```python
from build123d import *

# Parameters (mm, degrees)
SKETCH1_R           = 2.0828
SKETCH1_R_2         = 14.2875
SKETCH1_R_3         = 2.4892
BOSS_EXTRUDE1_DEPTH = 6.35


with BuildPart() as part:
    # Sketch1 → Boss-Extrude1 (new body)
    with BuildSketch(Plane(origin=(95.25, 0, 0), x_dir=(0, 0, -1), z_dir=(1, 0, 0))):
        with BuildLine():
            Line((-184.15, -107.95), (-184.15, -25.4))
            ThreePointArc((-184.15, -25.4), (-186.009871939, -20.909871939), (-190.5, -19.05))
            Line((-190.5, -19.05), (-215.9, -19.05))
            ThreePointArc((-215.9, -19.05), (-220.390128061, -20.909871939), (-222.25, -25.4))
            Line((-222.25, -25.4), (-222.25, -107.95))
            ThreePointArc((-222.25, -107.95), (-220.390128061, -112.440128061), (-215.9, -114.3))
            Line((-215.9, -114.3), (-190.5, -114.3))
            ThreePointArc((-190.5, -114.3), (-186.009871939, -112.440128061), (-184.15, -107.95))
        make_face()
        with Locations(Location((-190.376194259, -82.426194259, 0), (0, 0, 180))):
            Circle(SKETCH1_R, mode=Mode.SUBTRACT)
        with Locations(Location((-216.023805741, -108.073805741, 0), (0, 0, 180))):
            Circle(SKETCH1_R, mode=Mode.SUBTRACT)
        with Locations(Location((-203.2, -95.25, 0), (0, 0, 180))):
            Circle(SKETCH1_R_2, mode=Mode.SUBTRACT)
        with Locations(Location((-215.9, -31.75, 0), (0, 0, 180))):
            Circle(SKETCH1_R_3, mode=Mode.SUBTRACT)
        with Locations(Location((-203.2, -31.75, 0), (0, 0, 180))):
            Circle(SKETCH1_R_3, mode=Mode.SUBTRACT)
        with Locations(Location((-190.5, -31.75, 0), (0, 0, 180))):
            Circle(SKETCH1_R_3, mode=Mode.SUBTRACT)
        with Locations(Location((-215.9, -57.15, 0), (0, 0, 180))):
            Circle(SKETCH1_R_3, mode=Mode.SUBTRACT)
        with Locations(Location((-203.2, -57.15, 0), (0, 0, 180))):
            Circle(SKETCH1_R_3, mode=Mode.SUBTRACT)
        with Locations(Location((-190.5, -57.15, 0), (0, 0, 180))):
            Circle(SKETCH1_R_3, mode=Mode.SUBTRACT)
        with Locations(Location((-215.9, -44.45, 0), (0, 0, 180))):
            Circle(SKETCH1_R_3, mode=Mode.SUBTRACT)
        with Locations(Location((-203.2, -44.45, 0), (0, 0, 180))):
            Circle(SKETCH1_R_3, mode=Mode.SUBTRACT)
        with Locations(Location((-190.5, -44.45, 0), (0, 0, 180))):
            Circle(SKETCH1_R_3, mode=Mode.SUBTRACT)
    extrude(amount=-BOSS_EXTRUDE1_DEPTH)


solid = part.part
```
Part model, mm, in its own coordinate system. Coordinates: 2 decimals unless noted, no trailing zeros. Order: outer loops, then holes, each group sorted by start corner. A loop starts at its lowest first (then second) coordinate and runs counter-clockwise, first axis right, second up. Notation, with made-up numbers: (28.5, 67) -> (51.5, 67) arc R31 cw to (51.5, 91) -> close; hole circle Ø10 at (-12, 79). An arc over 180 degrees is marked (long way). Put each result on its own line as item: value. Start each with the question number.
(1) Band-saw the part on B-B (z = 209). Give the cut face in (x, y).
(2) Band-saw the part on D-D (y = -57.15). Give the cut face in (x, z), then the cut area to 3 significant figures.
(3) Band-saw the part on A-A (y = -95.25). Give the cut face in (x, z), then the cut area to 3 significant figures.
(4) Pin check, flat tip, straight feed: pin 1 Ø5.5 at (y, z) = (-57.15, 190.5) entering from +X. Stop position of the tip, or through.
(5) Probe line 1 along Y through (x, z) = (92.25, 203.2); line 2 along Z through (x, y) = (93, -44.5); line 3 along Z through (x, y) = (91, -44). List the from-to ranges inside material, lowest first. Write a range as [from, to].
(6) Band-saw the part on C-C (x = 89.75). Count the separate pieces of the cut face and the enclosed holes in it, then the cut area to 3 significant figures.
(7) Mould opens along Y. For faces 1 (the face through (92.1, -43.5, 205.5)), 2 (the face through (92.12, -20.96, 185.96)), 3 (the face through (95.25, -55, 199)) say: pulls with the +Y half, pulls with the -Y half, needs draft (parallel to the pull), parting line crosses it, or undercut.
Determined:
1. outline: (88.9, -114.3) -> (95.25, -114.3) -> (95.25, -108.31) -> (88.9, -108.31) -> close; (88.9, -82.19) -> (95.25, -82.19) -> (95.25, -19.05) -> (88.9, -19.05) -> close
2. outline: (88.9, 184.15) -> (95.25, 184.15) -> (95.25, 188.01) -> (88.9, 188.01) -> close; (88.9, 192.99) -> (95.25, 192.99) -> (95.25, 200.71) -> (88.9, 200.71) -> close; (88.9, 205.69) -> (95.25, 205.69) -> (95.25, 213.41) -> (88.9, 213.41) -> close; (88.9, 218.39) -> (95.25, 218.39) -> (95.25, 222.25) -> (88.9, 222.25) -> close
2. area: 147 mm²
3. outline: (88.9, 184.15) -> (95.25, 184.15) -> (95.25, 188.91) -> (88.9, 188.91) -> close; (88.9, 217.49) -> (95.25, 217.49) -> (95.25, 222.25) -> (88.9, 222.25) -> close
3. area: 60.5 mm²
4. pin 1: stops at x = 95.25
5. line 1: y = [-114.3, -109.54], [-80.96, -59.64], [-54.66, -46.94], [-41.96, -34.24], [-29.26, -19.05]
5. line 2: z = [184.15, 188.01], [192.99, 200.71], [205.69, 213.41], [218.39, 222.25]
5. line 3: z = [184.15, 188.05], [192.95, 200.75], [205.65, 213.45], [218.35, 222.25]
6. separate pieces: 1
6. enclosed holes: 12
6. area: 2,750 mm²
7. face 1: undercut
7. face 2: pulls with the +Y half
7. face 3: needs draft
